from build123d import *

# Parameters (mm, degrees)
BOSS_EXTRUDE5_DEPTH = 5
SKETCH1_8_R         = 3.25
BOSS_EXTRUDE6_DEPTH = 45
FILLET3_R           = 5
FILLET4_R           = 5
CUT_EXTRUDE1_DEPTH  = 45


with BuildPart() as part:
    # Sketch1 → Boss-Extrude5 (new body)
    # profile 1 of 4: a face of its own
    with BuildSketch(Plane(origin=(0, 0, 0), x_dir=(1, 0, 0), z_dir=(0, 1, 0))):
        with BuildLine():
            ThreePointArc((-82.5, 12.5), (-86.035533906, 11.035533906), (-87.5, 7.5))
            Line((-87.5, 7.5), (-87.5, -7.5))
            ThreePointArc((-87.5, -7.5), (-86.035533906, -11.035533906), (-82.5, -12.5))
            Line((-82.5, -12.5), (-43.229041164, -12.5))
            ThreePointArc((-43.229041164, -12.5), (-45, 0), (-43.229041164, 12.5))
            Line((-43.229041164, 12.5), (-82.5, 12.5))
        make_face()
        with BuildLine():
            ThreePointArc((-72.5, -2.5), (-75, 0), (-72.5, 2.5))
            Line((-72.5, 2.5), (-57.5, 2.5))
            ThreePointArc((-57.5, 2.5), (-55, 0), (-57.5, -2.5))
            Line((-57.5, -2.5), (-72.5, -2.5))
        make_face(mode=Mode.SUBTRACT)
    # profile 2 of 4: a face of its own
    with BuildSketch(Plane(origin=(0, 0, 0), x_dir=(1, 0, 0), z_dir=(0, 1, 0))):
        with BuildLine():
            Line((-37.996710384, 12.5), (-43.229041164, 12.5))
            ThreePointArc((-43.229041164, 12.5), (-45, 0), (-43.229041164, -12.5))
            Line((-43.229041164, -12.5), (-37.996710384, -12.5))
            ThreePointArc((-37.996710384, -12.5), (-40, 0), (-37.996710384, 12.5))
        make_face()
    # profile 3 of 4: a face of its own
    with BuildSketch(Plane(origin=(0, 0, 0), x_dir=(1, 0, 0), z_dir=(0, 1, 0))):
        with BuildLine():
            Line((43.229041164, 12.5), (37.996710384, 12.5))
            ThreePointArc((37.996710384, 12.5), (40, 0), (37.996710384, -12.5))
            Line((37.996710384, -12.5), (43.229041164, -12.5))
            ThreePointArc((43.229041164, -12.5), (45, 0), (43.229041164, 12.5))
        make_face()
    # profile 4 of 4: a face of its own
    with BuildSketch(Plane(origin=(0, 0, 0), x_dir=(1, 0, 0), z_dir=(0, 1, 0))):
        with BuildLine():
            Line((82.5, 12.5), (43.229041164, 12.5))
            ThreePointArc((43.229041164, 12.5), (45, 0), (43.229041164, -12.5))
            Line((43.229041164, -12.5), (82.5, -12.5))
            ThreePointArc((82.5, -12.5), (86.035533906, -11.035533906), (87.5, -7.5))
            Line((87.5, -7.5), (87.5, 7.5))
            ThreePointArc((87.5, 7.5), (86.035533906, 11.035533906), (82.5, 12.5))
        make_face()
        with BuildLine():
            ThreePointArc((72.5, 2.5), (75, 0), (72.5, -2.5))
            Line((72.5, -2.5), (57.5, -2.5))
            ThreePointArc((57.5, -2.5), (55, 0), (57.5, 2.5))
            Line((57.5, 2.5), (72.5, 2.5))
        make_face(mode=Mode.SUBTRACT)
    extrude(amount=BOSS_EXTRUDE5_DEPTH)

    # Sketch1_8 → Boss-Extrude6 (add)
    with BuildSketch(Plane(origin=(0, 0, 0), x_dir=(1, 0, 0), z_dir=(0, 1, 0))):
        with BuildLine():
            ThreePointArc((-37.996710384, 12.5), (-40, 0), (-37.996710384, -12.5))
            Line((-37.996710384, -12.5), (37.996710384, -12.5))
            ThreePointArc((37.996710384, -12.5), (40, 0), (37.996710384, 12.5))
            Line((37.996710384, 12.5), (-37.996710384, 12.5))
        make_face()
        with Locations(Location((-30.5, 0, 0), (0, 0, 90))):
            Circle(SKETCH1_8_R, mode=Mode.SUBTRACT)
        with Locations(Location((30.5, 0, 0), (0, 0, 90))):
            Circle(SKETCH1_8_R, mode=Mode.SUBTRACT)
    extrude(amount=BOSS_EXTRUDE6_DEPTH)

    # Fillet3
    fillet3_edges = [part.edges().sort_by_distance(p)[0] for p in [
        (-40, 5, 0),
    ]]
    fillet(fillet3_edges, radius=FILLET3_R)

    # Fillet4
    fillet4_edges = [part.edges().sort_by_distance(p)[0] for p in [
        (40, 5, 0),
    ]]
    fillet(fillet4_edges, radius=FILLET4_R)

    # Sketch4 → Cut-Extrude1 (cut)
    with BuildSketch(Plane.XY.offset(12.5)):
        with BuildLine():
            Line((-21.496710384, 45), (-21.496710384, 35))
            Line((-21.496710384, 35), (-18.496710384, 35))
            ThreePointArc((-18.496710384, 35), (0.003289616, 16.5), (18.503289616, 35))
            Line((18.503289616, 35), (21.503289616, 35))
            Line((21.503289616, 35), (21.503289616, 45))
            Line((21.503289616, 45), (-21.496710384, 45))
        make_face()
    extrude(amount=-CUT_EXTRUDE1_DEPTH, mode=Mode.SUBTRACT)


solid = part.part
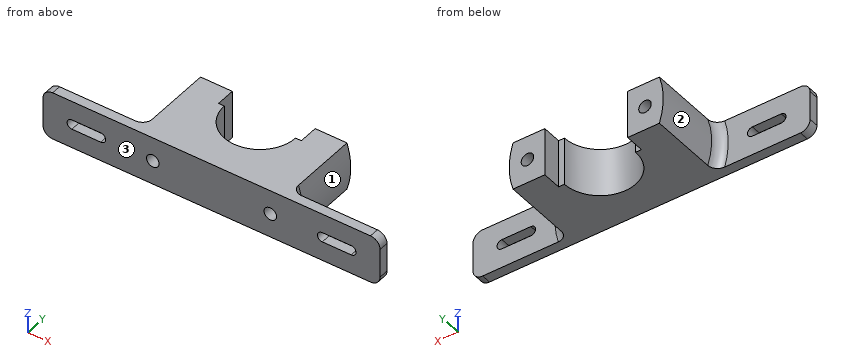
Design review of the part built by this model. Coordinates are the model's own, in mm. Face numbers are marked on the shaded views. A direction names the side the tool comes from. Coordinates: 2 decimals unless noted, no trailing zeros. Loops run counter-clockwise (first coordinate to the right, second up) from the corner with the lowest first, then second, coordinate; pieces in that order, holes last. Notation, with made-up numbers: M -34,12.5 L 17,12.5 A17 cw 17,28.5 Z; hole C 61,-35.5 d2. An arc over 180 degrees is marked long. Use one line per item in the form item = value.
(1) Clearance check with flat-ended pins moving along their axes: P1, Ø2.5, axis at x = 20, z = -0.5, coming from the +Y side; P2, Ø5, axis at y = 41, z = -0.5, coming from the +X side; P3, Ø6, axis at y = 31, z = 4, coming from the -X side. State where each tip first meets the part, or that it passes through.
Return value:
P1 = 35
P2 = 40
P3 = -39.99
(2) For the marked faces 1, 2 and 3, list the 3-axis set-ups (+Z, -Z, +X, -X, +Y, -Y) from which the entire face can be reached by the end or side of a thin tool; tool diameter is ignored.
Return value:
face_1 = +X, +Y
face_2 = -X, +Y
face_3 = +Z, -Z, +X, -X, -Y
(3) Consider section B-B (x = -30.5). Write out the cut boundary in (y, z), and give its area (4 significant figures).
Return value:
outline = M 0,-12.5 L 45,-12.5 L 45,-3.25 L 0,-3.25 Z; M 0,3.25 L 45,3.25 L 45,12.5 L 0,12.5 Z
area = 832.5 mm2
(4) Consider section A-A (z = 0). Give the number of separate pieces and of enclosed holes in the cut face, and give its area (3 significant figures).
Return value:
separate_pieces = 5
enclosed_holes = 0
area = 2,330 mm2
(5) For line 1 along Z through (x, y) = (30.5, 30.5); line 2 along X through (y, z) = (25, -1.25); line 3 along Y through (x, z) = (-68, -8.5), list the stretches that pass through material, from the lowest coordinate up. Write a range as from..to.
Return value:
line_1 = -12.5..-3.25, 3.25..12.5
line_2 = -39.98..-33.5, -27.5..-15.56, 15.57..27.5, 33.5..39.98
line_3 = 0..5
(6) Consider section D-D (x = 6). Write out the cut boundary in (y, z).
Return value:
outline = M 0,-12.5 L 17.5,-12.5 L 17.5,12.5 L 0,12.5 Z
(7) Consider section C-C (y = 3). Write out the cut boundary in (x, z), and give its area (3 significant figures).
Return value:
outline = M -87.5,-7.5 A5 ccw -82.5,-12.5 L 82.5,-12.5 A5 ccw 87.5,-7.5 L 87.5,7.5 A5 ccw 82.5,12.5 L -82.5,12.5 A5 ccw -87.5,7.5 Z; hole M -72.5,-2.5 L -57.5,-2.5 A2.5 ccw -57.5,2.5 L -72.5,2.5 A2.5 ccw Z; hole C -30.5,0 d6.5; hole C 30.5,0 d6.5; hole M 57.5,-2.5 L 72.5,-2.5 A2.5 ccw 72.5,2.5 L 57.5,2.5 A2.5 ccw Z
area = 4,100 mm2
